Verification items for this drawing (mm, ordinates from the low corner). A direction names the side the tool comes from. Round coordinates to 2 decimals unless told otherwise and drop trailing zeros. Loops run counter-clockwise (first coordinate to the right, second up) from the corner with the lowest first, then second, coordinate; pieces in that order, holes last. Notation, with made-up numbers: (65.5, -35) - (75.5, -35) arc R27 cw to (75.5, -4) - close; hole circle Ø2 at (19, 32). An arc over 180 degrees is marked (long way). Write item = value, one per line.
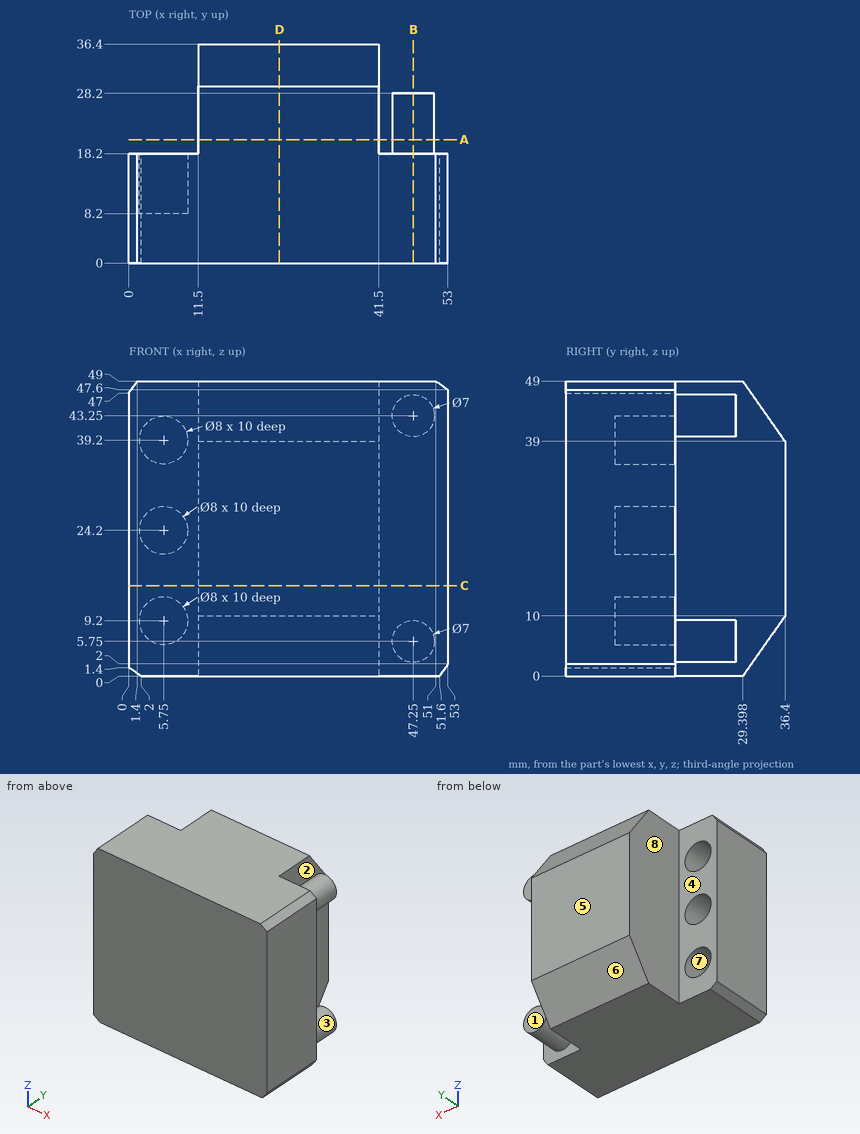
(1) Section check C-C (z = 15). Enter the section's corners in (x, y).
Answers follow:
outline = (0, 0) - (53, 0) - (53, 18.2) - (41.5, 18.2) - (41.5, 36.4) - (11.5, 36.4) - (11.5, 18.2) - (0, 18.2) - close
(2) Section check A-A (y = 20.5). Enter the section's corners in (x, z).
Answers follow:
outline = (11.5, 0) - (41.5, 0) - (41.5, 49) - (11.5, 49) - close; circle Ø7 at (47.25, 5.75); circle Ø7 at (47.25, 43.25)
(3) Mould release check, pull along X, two halves, no side actions. Record for the marked faces 6, 7 and 8: pulls with the +X half, pulls with the -X half, needs draft (parallel to the pull), parting line crosses it, or undercut.
Answers follow:
face_6 = needs draft
face_7 = undercut
face_8 = pulls with the -X half
(4) Section check D-D (x = 25). Enter the section's corners in (y, z), then the cut area to 3 significant figures.
Answers follow:
outline = (0, 0) - (29.4, 0) - (36.4, 10) - (36.4, 39) - (29.4, 49) - (0, 49) - close
area = 1,710 mm²
(5) Gauge pin test, flat ends, axial feed: pin 1 (6.5 mm diameter, centred on x = 7.5, z = 10.5, fed in from +Y); pin 2 (7.5 mm diameter, centred on x = 47, z = 6, fed in from +Y); pin 3 (14.5 mm diameter, centred on y = 30, z = 35, fed in from -X). Record the tip position at first contact, or that the pin passes through.
Answers follow:
pin_1 = 18.2
pin_2 = 28.2
pin_3 = 11.5
(6) Scan lines: L1, parallel to Z at x = 5.75, y = 13.5; L2, parallel to X at y = 22.5, z = 13; L3, parallel to Y at x = 3.5, z = 7.5. Record each from-to range of solid material in increasing order. Write a range as [from, to].
Answers follow:
L1 = [0, 5.2], [13.2, 20.2], [28.2, 35.2], [43.2, 49]
L2 = [11.5, 41.5]
L3 = [0, 8.2]
(7) Set-up check for the marked faces 1, 2, 3, 4 and 5: record each of +Z, -Z, +X, -X, +Y, -Y from which the full face is reachable in a straight line by a thin tool's end or side.
Answers follow:
face_1 = +Z, -Z, +X, +Y
face_2 = +Z, -Z, +Y
face_3 = +Y
face_4 = +Z, -Z, -X, +Y
face_5 = +Z, -Z, +X, -X, +Y
(8) Section check B-B (x = 47.25). Enter the section's corners in (y, z).
Answers follow:
outline = (0, 0) - (18.2, 0) - (18.2, 2.25) - (28.2, 2.25) - (28.2, 9.25) - (18.2, 9.25) - (18.2, 39.75) - (28.2, 39.75) - (28.2, 46.75) - (18.2, 46.75) - (18.2, 49) - (0, 49) - close
